Read the model definition and answer for the solid it produces. Units are mm, in the model's axes. Give positions to 0.01 mm unless a question says otherwise; leave off trailing zeros. Order: outer loops, then holes, each group sorted by start corner. A loop starts at its lowest first (then second) coordinate and runs counter-clockwise, first axis right, second up. Notation, with made-up numbers: (13, 53) - (33, 53) arc R9 ccw to (33, 62) - close; hole circle Ø10 at (14, -15). An arc over 180 degrees is marked (long way). Use a Markdown table: item, result. Add a question column.
1. A cutting plane is placed at A-A on y = -2.5. Determine the outline of the cut face in (x, z), and give its area (3 significant figures).
2. A cutting plane is placed at B-B on z = -4.5. Determine the outline of the cut face in (x, y).
3. Flat-ended cylindrical pins translate along their axes: P1, Ø2, axis at y = 3, z = -11, coming from the +X side; P2, Ø6, axis at y = -1.5, z = -9.5, coming from the -X side; P3, Ø4, axis at y = 0, z = -7, coming from the -X side. Find the tip coordinate at first contact, or state that the pin passes through.
4. For a pull along Z with two mould halves and no side action, classify faces 1 (the cylindrical face through (-14.609, 0.07, -9.536)), 2 (the cylindrical face through (34.632, -0.346, -9.881)), 3 (the flat face through (-42.13, -0.07, -8)), 4 (the flat face through (-2, -5, -8)) as released by +Z, released by -Z, zero draft, split by the parting line, or undercut.
5. Consider L1, parallel to X at y = -2, z = -8.25; L2, parallel to X at y = -2.25, z = -8.75; L3, parallel to Z at x = 10, y = -1. Determine where each line is inside the solid, lowest interval first.
```python
from build123d import *

# Parameters (mm, degrees)
F0_R     = 1.5
F0_R_2   = 1.25
F1_DEPTH = 5
F3_D     = 1.5
F3_DEPTH = 5
F3_TIP   = 0.4506454643


with BuildPart() as f1:
    # F0 (on Front) → F1 (new body, symmetric)
    with BuildSketch(Plane.XZ):
        Polygon((35.7166262344, -3.072109893), (-39.2833737656, -3.072109893), (-45.0568764575, -13.072109893), (-39.2833737656, -13.072109893), (35.7166262344, -13.072109893), (41.4901289262, -3.072109893), align=None)
        with Locations((-14.2833737656, -8.072109893)):
            Circle(F0_R, mode=Mode.SUBTRACT)
        with Locations((10.7166262344, -8.072109893)):
            Circle(F0_R_2, mode=Mode.SUBTRACT)
    extrude(amount=F1_DEPTH, both=True)

    # F3
    with Locations(Plane(origin=(32.4478592999, 0, -18.7337803015), x_dir=(0, 1, 0), z_dir=(0.8660254038, 0, -0.5))):
        with Locations((0, 9.4242852148)):
            Hole(F3_D / 2, depth=F3_DEPTH)
            with Locations((0, 0, -(F3_DEPTH + F3_TIP / 2))):  # 118° drill point
                Cone(0, F3_D / 2, F3_TIP, mode=Mode.SUBTRACT)


solid = f1.part
```
Output values:
| question | item | result |
|---|---|---|
| 1 | outline | (-45.06, -13.07) - (35.72, -13.07) - (41.49, -3.07) - (-39.28, -3.07) - close; hole circle Ø3 at (-14.28, -8.07); hole circle Ø2.5 at (10.72, -8.07) |
| 1 | area | 796 mm² |
| 2 | outline | (-40.11, -5) - (40.67, -5) - (40.67, 5) - (-40.11, 5) - close |
| 3 | P1 | x = 37.49 |
| 3 | P2 | x = -44.73 |
| 3 | P3 | x = -42.71 |
| 4 | face 1 | undercut |
| 4 | face 2 | undercut |
| 4 | face 3 | released by +Z |
| 4 | face 4 | zero draft |
| 5 | L1 | -42.27 to -15.77, -12.79 to 9.48, 11.95 to 38.5 |
| 5 | L2 | -42.56 to -15.62, -12.95 to 9.67, 11.77 to 38.21 |
| 5 | L3 | -13.07 to -9.1, -7.05 to -3.07 |
